from build123d import *

# Parameters (mm, degrees)
BOSS_EXTRUDE1_DEPTH = 3.175
SKETCH2_R           = 7.14375
SKETCH2_R_2         = 3.175
CUT_EXTRUDE1_DEPTH  = 421.832566498


with BuildPart() as part:
    # Sketch1 → Boss-Extrude1 (new body)
    with BuildSketch(Plane(origin=(0, 0, 0), x_dir=(1, 0, 0), z_dir=(0, 1, 0))):
        Polygon((0, 0), (406.4, 0), (406.4, 41.275), (161.29, 41.275), (161.29, 109.22), (59.69, 109.22), (59.69, 41.275), (0, 41.275), align=None)
    extrude(amount=BOSS_EXTRUDE1_DEPTH)

    # Sketch2 → Cut-Extrude1 (cut, through all)
    with BuildSketch(Plane(origin=(0, 3.175, 0), x_dir=(1, 0, 0), z_dir=(0, 1, 0))):
        with Locations(Location((28.575, 20.6375, 0), (0, 0, 270))):
            Circle(SKETCH2_R)
        with Locations(Location((72.39, 90.17, 0), (0, 0, 270))):
            Circle(SKETCH2_R_2)
        with Locations(Location((330.2, 20.6375, 0), (0, 0, 270))):
            Circle(SKETCH2_R)
        with Locations(Location((377.825, 20.6375, 0), (0, 0, 270))):
            Circle(SKETCH2_R)
        with Locations(Location((72.39, 39.37, 0), (0, 0, 270))):
            Circle(SKETCH2_R_2)
        with Locations(Location((148.59, 39.37, 0), (0, 0, 270))):
            Circle(SKETCH2_R_2)
        with Locations(Location((148.59, 90.17, 0), (0, 0, 270))):
            Circle(SKETCH2_R_2)
    extrude(amount=-CUT_EXTRUDE1_DEPTH, mode=Mode.SUBTRACT)


solid = part.part
Model file for the job. Use its own axes, mm. Give positions to 0.01 mm unless a question says otherwise; leave off trailing zeros. Order: outer loops, then holes, each group sorted by start corner. A loop starts at its lowest first (then second) coordinate and runs counter-clockwise, first axis right, second up. Notation, with made-up numbers: (45, 48) - (51, 48) arc R27 ccw to (51, 72) - close; hole circle Ø7 at (-33, 55). An arc over 180 degrees is marked (long way). One line per item, written item: value.
Item 1: Wall check: line 1 (Z direction, x = 149, y = 0.2); line 2 (X direction, y = 0.9, z = -39.37) (3 decimals); line 3 (X direction, y = 2.25, z = -90.17) (3 decimals). Give the ranges that are in metal, low to high.
Response values:
line 1: -109.22 to -93.32, -87.02 to -42.52, -36.22 to 0
line 2: 0 to 69.215, 75.565 to 145.415, 151.765 to 406.4
line 3: 59.69 to 69.215, 75.565 to 145.415, 151.765 to 161.29
Item 2: Slice it at B-B (z = -17.5). List the corners of the cut face in (x, y) (3 decimals), then the cut area to 3 significant figures.
Response values:
outline: (0, 0) - (22.157, 0) - (22.157, 3.175) - (0, 3.175) - close; (34.993, 0) - (323.782, 0) - (323.782, 3.175) - (34.993, 3.175) - close; (336.618, 0) - (371.407, 0) - (371.407, 3.175) - (336.618, 3.175) - close; (384.243, 0) - (406.4, 0) - (406.4, 3.175) - (384.243, 3.175) - close
area: 1,170 mm2
Item 3: Slice it at C-C (y = 1.6). Give the number of separate pieces and of enclosed holes in the cut face, then the cut area to 3 significant figures.
Response values:
separate pieces: 1
enclosed holes: 7
area: 23,100 mm2
Item 4: Slice it at D-D (z = -76). List the corners of the cut face in (x, y) (3 decimals).
Response values:
outline: (59.69, 0) - (161.29, 0) - (161.29, 3.175) - (59.69, 3.175) - close
Item 5: Slice it at A-A (x = 330.2). List the corners of the cut face in (y, z) (3 decimals), then the cut area to 3 significant figures.
Response values:
outline: (0, -41.275) - (3.175, -41.275) - (3.175, -27.781) - (0, -27.781) - close; (0, -13.494) - (3.175, -13.494) - (3.175, 0) - (0, 0) - close
area: 85.7 mm2
Item 6: Pin check, flat tips, straight feed: pin 1 Ø18.5 at (x, z) = (330.2, -20.64) entering from +Y (3 decimals); pin 2 Ø5 at (x, z) = (148.59, -90.17) entering from -Y; pin 3 Ø1.6 at (y, z) = (1.5, -90.5) entering from -X; pin 4 Ø1.5 at (y, z) = (2.5, -74.5) entering from +X. Stop position of each tip, or through.
Response values:
pin 1: y = 3.175
pin 2: through
pin 3: x = 59.69
pin 4: x = 161.29
Item 7: Two-plate mould, pull along X, no slides. Class faces 1 (the cylindrical face through (145.5, 1.6, -40.1)), 2 (the flat face through (155, 3.175, -43)): released by +X, released by -X, zero draft, split by the parting line, or undercut.
Response values:
face 1: undercut
face 2: zero draft
